Can you work these out from the model? Positions are in its coordinate system, mm. Face numbers are marked on the shaded views. Give positions to 0.01 mm unless a question says otherwise; leave off trailing zeros. Write each loop counter-clockwise with the first axis right and the second up, starting at its lowest first coordinate (ties: lowest second). Pieces come first, ordered by that corner, then holes.
from build123d import *

# Parameters (mm, degrees)
SKETCH3_R          = 1.016
CUT_EXTRUDE1_DEPTH = 7.5
CIRPATTERN1_COUNT  = 6


with BuildPart() as part:
    # Sketch1 → Revolve1 (revolve)
    with BuildSketch(Plane(origin=(0, 0, 0), x_dir=(0, 0, -1), z_dir=(1, 0, 0))):
        with BuildLine():
            Line((3.175, 6.5), (14.483287783, 6.5))
            ThreePointArc((14.483287783, 6.5), (15.875, 0), (14.483287783, -6.5))
            Line((14.483287783, -6.5), (3.175, -6.5))
            Line((3.175, -6.5), (3.175, 6.5))
        make_face()
    revolve(axis=Axis((0, -6.5, 0), (0, 1, 0)))

    # Sketch3 → Cut-Extrude1 (cut, symmetric)
    with BuildSketch(Plane(origin=(0, 0, 0), x_dir=(1, 0, 0), z_dir=(0, 1, 0))):
        with Locations((7.9375, 0)):
            Circle(SKETCH3_R)
    cut_extrude1 = extrude(amount=CUT_EXTRUDE1_DEPTH, both=True, mode=Mode.SUBTRACT)

    # CirPattern1: Cut-Extrude1 ×6 about axis
    cirpattern1_axis = Axis((0, 0, 0), (0, 1, 0))
    for i in range(1, CIRPATTERN1_COUNT):
        add(cut_extrude1.rotate(cirpattern1_axis, i * 360 / CIRPATTERN1_COUNT), mode=Mode.SUBTRACT)


solid = part.part
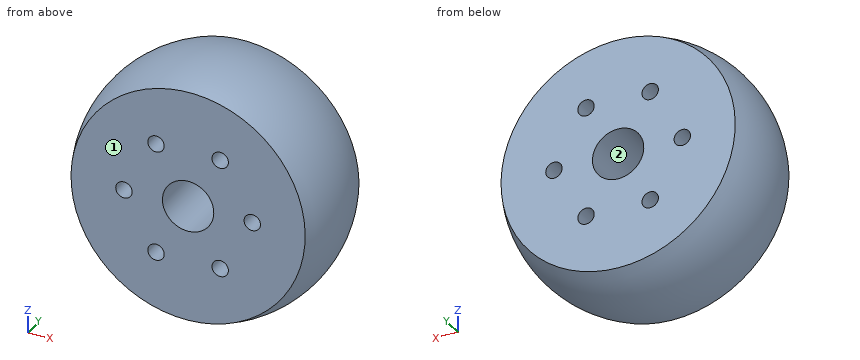
(1) If I drill on L1, parallel to Z at x = 2, y = -4.5; L2, parallel to X at y = 0.25, z = -2.5; L3, parallel to Z at x = 11.5, y = -5, over which ranges is the centre line in solid material (lowest first)?
Returned:
L1: z = -15.09 to -2.47, 2.47 to 15.09
L2: x = -15.67 to -1.96, 1.96 to 15.67
L3: z = -9.73 to 9.73
(2) Imagine slicing it at B-B, the plane z = 0. Give the number of separate pieces and of enclosed holes in the cut face, plus the area to 3 significant figures.
Returned:
separate pieces: 4
enclosed holes: 0
area: 266 mm2
(3) Will these pins go through, and if not, where does the flat tip stop? P1, Ø6, axis at x = 5, y = -3, coming from the +Z side; P2, Ø2, axis at y = 1, z = -10.5, coming from the +X side; P3, Ø1.5, axis at y = -2.5, z = -8.5, coming from the +X side.
Returned:
P1: stops at z = 15.62
P2: stops at x = 12.68
P3: stops at x = 13.65
(4) Imagine slicing it at A-A, the plane x = 0. Write out the boundary of the cut face in (y, z) (3 decimals).
Returned:
outline: (-6.5, -14.483) arc R15.875 ccw to (6.5, -14.483) - (6.5, -3.175) - (-6.5, -3.175) - close; (-6.5, 3.175) - (6.5, 3.175) - (6.5, 14.483) arc R15.875 ccw to (-6.5, 14.483) - close
(5) If we mould it in two halves opening along X, with no side actions, what happens to the marked faces 1 and 2? For each: +X half, -X half, draft (parallel to the pull), parting line (faces both ways), or undercut.
Returned:
face 1: draft
face 2: undercut
